from build123d import *

# Parameters (mm, degrees)
SKETCH2_R                  = 5.5499
BOSS_EXTRUDE1_DEPTH        = 3.175
CUT_EXTRUDE1_DEPTH         = 3.175
CUT_EXTRUDE6_DEPTH         = 331.886967859
CUT_EXTRUDE6_DEPTH_BACK    = 331.886967859
SKETCH32_R                 = 2.38125
CUT_EXTRUDE4_DEPTH         = 331.886967859
F_1_1_DIAMETER_HOLE1_D     = 31.75
F_8_CLEARANCE_HOLE1_D      = 4.4958
FILLET1_R                  = 25.4
FILLET2_R                  = 6.35
CUT_EXTRUDE7_START         = -1.74625
SKETCH34_R                 = 3.968749998
SKETCH34_R_2               = 3.96875
SKETCH34_R_3               = 3.968749996
CUT_EXTRUDE7_DEPTH         = 1.74625
F_8_0_199_DIAMETER_HOLE1_D = 5.0546
CUT_EXTRUDE9_DEPTH         = 331.886967859


with BuildPart() as part:
    # Sketch2 → Boss-Extrude1 (new, symmetric)
    with BuildSketch(Plane(origin=(0, 0, 0), x_dir=(0, 0, -1), z_dir=(1, 0, 0))):
        with BuildLine():
            Line((184.861603477, 125.395219788), (192.888179376, 122.398060471))
            ThreePointArc((192.888179376, 122.398060471), (197.134402772, 119.670037319), (199.868014027, 115.427409246))
            ThreePointArc((199.868014027, 115.427409246), (205.79135088, 101.944347228), (213.165326628, 89.196666555))
            ThreePointArc((213.165326628, 89.196666555), (245.495612564, 46.296629776), (283.201634595, 8.035468699))
            ThreePointArc((283.201634595, 8.035468699), (289.498729419, -0.543862964), (291.728224202, -10.95))
            Line((291.728224202, -10.95), (291.728224202, -63.147045251))
            ThreePointArc((291.728224202, -63.147045251), (290.86274019, -69.721048996), (288.325269458, -75.847045251))
            Line((288.325269458, -75.847045251), (279.028224202, -91.949999995))
            Line((279.028224202, -91.949999995), (258.619227522, -91.949999995))
            ThreePointArc((258.619227522, -91.949999995), (257.031727522, -90.362499995), (255.444227522, -91.949999995))
            Line((255.444227522, -91.949999995), (255.444227522, -98.3))
            Line((255.444227522, -98.3), (230.044227522, -98.3))
            Line((230.044227522, -98.3), (230.044227522, -91.949999995))
            ThreePointArc((230.044227522, -91.949999995), (228.456727522, -90.362499995), (226.869227522, -91.949999995))
            Line((226.869227522, -91.949999995), (206.460230842, -91.949999995))
            ThreePointArc((206.460230842, -91.949999995), (203.285230842, -88.774999995), (200.110230842, -91.949999995))
            Line((200.110230842, -91.949999995), (200.110230842, -110.516313332))
            ThreePointArc((200.110230842, -110.516313332), (188.495902289, -129.333888909), (175.117759697, -146.941247574))
            ThreePointArc((175.117759697, -146.941247574), (139.333425556, -150.071971144), (136.202701987, -114.287637002))
            ThreePointArc((136.202701987, -114.287637002), (177.123417321, -15.496291061), (153.979316793, 88.9))
            ThreePointArc((153.979316793, 88.9), (156.586799992, 118.007464254), (184.861603477, 125.395219788))
        make_face()
        with Locations((188.725443767, 111.25)):
            Circle(SKETCH2_R, mode=Mode.SUBTRACT)
    extrude(amount=BOSS_EXTRUDE1_DEPTH, both=True)

    # Sketch4 → Cut-Extrude1 (cut)
    with BuildSketch(Plane.ZY.offset(3.175)):
        with BuildLine():
            ThreePointArc((-142.891227531, -119.899976319), (-139.536446205, -120.193481654), (-139.24294087, -116.838700328))
            ThreePointArc((-139.24294087, -116.838700328), (-180.470281158, -21.687694559), (-162.960405636, 80.521951489))
            ThreePointArc((-162.960405636, 80.521951489), (-164.040385384, 83.711676692), (-167.230110587, 82.631696943))
            ThreePointArc((-167.230110587, 82.631696943), (-185.19876014, -22.255931098), (-142.891227531, -119.899976319))
        make_face()
    extrude(amount=-CUT_EXTRUDE1_DEPTH, mode=Mode.SUBTRACT)

    # Sketch32 → Cut-Extrude6 (cut, two sides: drawn at the far end of the back side and taken through both)
    with BuildSketch(Plane.ZY.offset(3.175).offset(-CUT_EXTRUDE6_DEPTH_BACK)):
        with Locations((-159.478578107, 92.075)):
            Circle(SKETCH32_R)
    extrude(amount=CUT_EXTRUDE6_DEPTH + CUT_EXTRUDE6_DEPTH_BACK, mode=Mode.SUBTRACT)

    # Sketch23 → Cut-Extrude4 (cut, through all)
    with BuildSketch(Plane(origin=(3.175, 0, 0), x_dir=(0, 0, -1), z_dir=(1, 0, 0))):
        with BuildLine():
            Line((191.834020078, -91.95), (191.834020078, -98.3))
            ThreePointArc((191.834020078, -98.3), (190.246520078, -99.8875), (188.659020078, -98.3))
            Line((188.659020078, -98.3), (175.959020078, -98.3))
            ThreePointArc((175.959020078, -98.3), (174.371520078, -99.8875), (172.784020078, -98.3))
            Line((172.784020078, -98.3), (172.784020078, -91.95))
            ThreePointArc((172.784020078, -91.95), (174.371520078, -90.3625), (175.959020078, -91.95))
            Line((175.959020078, -91.95), (188.659020078, -91.95))
            ThreePointArc((188.659020078, -91.95), (190.246520078, -90.3625), (191.834020078, -91.95))
        make_face()
    extrude(amount=-CUT_EXTRUDE4_DEPTH, mode=Mode.SUBTRACT)

    # 1 (1) Diameter Hole1 (through all)
    with Locations(Plane(origin=(3.175, 0, 0), x_dir=(0, 0, -1), z_dir=(1, 0, 0))):
        with Locations((255.178224202, -28.45)):
            Hole(F_1_1_DIAMETER_HOLE1_D / 2)

    # #8 Clearance Hole1 (through all)
    with Locations(Plane.ZY.offset(3.175)):
        with Locations((-273.138736444, -46.410512242), (-237.21771196, -10.489487758)):
            Hole(F_8_CLEARANCE_HOLE1_D / 2)

    # Fillet1
    fillet1_edges = [part.edges().sort_by_distance(p)[0] for p in [
        (0, -110.516313332, -200.110230842),
    ]]
    fillet(fillet1_edges, radius=FILLET1_R)

    # Fillet2
    fillet2_edges = [part.edges().sort_by_distance(p)[0] for p in [
        (0, -91.949999995, -206.460230842),
    ]]
    fillet(fillet2_edges, radius=FILLET2_R)

    # Sketch34 → Cut-Extrude7 (cut)
    with BuildSketch(Plane.ZY.offset(3.175).offset(CUT_EXTRUDE7_START)):
        with Locations((-272.678224202, -72.899999995)):
            Circle(SKETCH34_R)
        with Locations((-272.678224202, 3.300000005)):
            Circle(SKETCH34_R)
        with Locations((-209.953929472, -72.899999995)):
            Circle(SKETCH34_R_2)
        with Locations((-221.091752478, 22.660527049)):
            Circle(SKETCH34_R)
        with Locations((-200.007931611, 96.911762922)):
            Circle(SKETCH34_R_3)
        with Locations((-152.402488977, -139.565014501)):
            Circle(SKETCH34_R_2)
    extrude(amount=CUT_EXTRUDE7_DEPTH, mode=Mode.SUBTRACT)

    # #8 (0.199) Diameter Hole1 (through all)
    with Locations(Plane(origin=(3.175, 0, 0), x_dir=(0, 0, -1), z_dir=(1, 0, 0))):
        with Locations((272.678224202, -72.899999995), (209.953929472, -72.899999995), (221.091752478, 22.660527049), (200.007931611, 96.911762922), (272.678224202, 3.300000005), (152.402488977, -139.565014501)):
            Hole(F_8_0_199_DIAMETER_HOLE1_D / 2)

    # Sketch38 → Cut-Extrude9 (cut, through all)
    with BuildSketch(Plane(origin=(3.175, 0, 0), x_dir=(0, 0, -1), z_dir=(1, 0, 0))):
        with BuildLine():
            Line((205.914798647, 28.562805507), (224.924360785, 39.537981324))
            ThreePointArc((224.924360785, 39.537981324), (227.99131211, 43.870819192), (226.69603004, 49.018820627))
            ThreePointArc((226.69603004, 49.018820627), (214.944800076, 64.327050851), (203.910748393, 80.160023463))
            ThreePointArc((203.910748393, 80.160023463), (190.936466062, 83.542932982), (186.142659774, 71.021131989))
            ThreePointArc((186.142659774, 71.021131989), (192.251844092, 52.271592857), (196.477565484, 33.009956649))
            ThreePointArc((196.477565484, 33.009956649), (200.032947992, 28.317899385), (205.914798647, 28.562805507))
        make_face()
        with BuildLine():
            Line((205.310000647, -4.207176979), (211.8854012, -4.207176979))
            ThreePointArc((211.8854012, -4.207176979), (216.375529261, -6.067048919), (218.2354012, -10.557176979))
            Line((218.2354012, -10.557176979), (218.2354012, -46.34282301))
            ThreePointArc((218.2354012, -46.34282301), (216.375529261, -50.832951071), (211.8854012, -52.69282301))
            Line((211.8854012, -52.69282301), (200.289772847, -52.69282301))
            ThreePointArc((200.289772847, -52.69282301), (195.319253016, -50.294586238), (194.103216157, -44.911384462))
            ThreePointArc((194.103216157, -44.911384462), (197.299266335, -27.67833955), (198.968379006, -10.23108657))
            ThreePointArc((198.968379006, -10.23108657), (200.936682347, -5.953201844), (205.310000647, -4.207176979))
        make_face()
        with BuildLine():
            Line((229.003929472, -65.39282301), (253.628224202, -65.39282301))
            ThreePointArc((253.628224202, -65.39282301), (258.118352263, -67.25269495), (259.978224202, -71.74282301))
            Line((259.978224202, -71.74282301), (259.978224202, -72.899999995))
            ThreePointArc((259.978224202, -72.899999995), (258.118352263, -77.390128055), (253.628224202, -79.249999995))
            Line((253.628224202, -79.249999995), (229.003929472, -79.249999995))
            ThreePointArc((229.003929472, -79.249999995), (224.513801412, -77.390128055), (222.653929472, -72.899999995))
            Line((222.653929472, -72.899999995), (222.653929472, -71.74282301))
            ThreePointArc((222.653929472, -71.74282301), (224.513801412, -67.25269495), (229.003929472, -65.39282301))
        make_face()
        with BuildLine():
            Line((178.614385619, -107.825), (163.596957108, -107.825))
            ThreePointArc((163.596957108, -107.825), (157.868812502, -109.190170518), (153.372147289, -112.9921875))
            ThreePointArc((153.372147289, -112.9921875), (151.919142792, -114.938348924), (150.441444733, -116.865827797))
            ThreePointArc((150.441444733, -116.865827797), (149.54669032, -123.085290269), (154.438269364, -127.02924176))
            ThreePointArc((154.438269364, -127.02924176), (158.545587593, -128.449604505), (161.93353243, -131.171611694))
            ThreePointArc((161.93353243, -131.171611694), (166.924642658, -133.320901925), (171.750540646, -130.822634844))
            ThreePointArc((171.750540646, -130.822634844), (177.370609198, -123.095397934), (182.643281535, -115.127067669))
            ThreePointArc((182.643281535, -115.127067669), (182.784283536, -110.2867702), (178.614385619, -107.825))
        make_face()
        with BuildLine():
            ThreePointArc((229.352144485, 13.013977205), (232.770157357, 17.670050169), (233.772565242, 23.358372055))
            ThreePointArc((233.772565242, 23.358372055), (237.643482483, 29.557433307), (244.785557135, 28.00722998))
            ThreePointArc((244.785557135, 28.00722998), (250.350507009, 22.07652944), (256.029490766, 16.254930046))
            ThreePointArc((256.029490766, 16.254930046), (257.782536544, 10.684174236), (254.244609375, 6.037717399))
            ThreePointArc((254.244609375, 6.037717399), (245.943574881, 3.17910276), (237.21771196, 2.210512242))
            ThreePointArc((237.21771196, 2.210512242), (235.966501016, 2.148726957), (234.727464312, 1.96397227))
            ThreePointArc((234.727464312, 1.96397227), (227.77212485, 5.41294467), (229.352144485, 13.013977205))
        make_face()
    extrude(amount=-CUT_EXTRUDE9_DEPTH, mode=Mode.SUBTRACT)


solid = part.part
Source: CAD feature listing. Evaluate the final solid. Frame: model axes, mm. A direction names the side the tool comes from. Round coordinates to 2 decimals unless told otherwise and drop trailing zeros. Order: outer loops, then holes, each group sorted by start corner. A loop starts at its lowest first (then second) coordinate and runs counter-clockwise, first axis right, second up. Notation, with made-up numbers: (74, -33) -> (92, -33) arc R15 cw to (92, -29) -> close; hole circle Ø4 at (0.25, -37.5). An arc over 180 degrees is marked (long way). Answer as CSV lines item,"result".
Item 1: Section D-D, the plane x = 2. Count the separate pieces of the cut face and the enclosed holes in it, plus the area to 3 significant figures.
A:
separate pieces,"1"
enclosed holes,"17"
area,"18,000 mm²"
Item 2: Section C-C, the plane y = 111.25. Return loops of the section in (x, z) (3 decimals), plus the area to 3 significant figures.
A:
outline,"(-3.175, -201.515) -> (3.175, -201.515) -> (3.175, -194.275) -> (-3.175, -194.275) -> close; (-3.175, -183.176) -> (3.175, -183.176) -> (3.175, -152.481) -> (-3.175, -152.481) -> close"
area,"241 mm²"
Item 3: Line query: L1, parallel to Y at x = -1.75, z = -226; L2, parallel to Y at x = 0.75, z = -153; L3, parallel to Y at x = 3, z = -241. Output: solid intervals per line, ascending.
A:
L1,"-91.95 to -78.49, -66.15 to 40.32, 49.89 to 70.73"
L2,"-155.87 to -142.02, -137.11 to -126.62, -113.5 to -90.58, 90.77 to 112.43"
L3,"-98.3 to -79.25, -65.39 to -35.59, -21.31 to 2.39, 30 to 51.6"
Item 4: Reachability of faces 4 (the face through (0.04, 46.87, -245)), 5 (the face through (0.04, -77.34, -258.17)), 6 (the face through (-2.29, -71.71, -268.89)) from +Z, -Z, +X, -X, +Y, -Y: full face, straight path, thin tool, end or side. Return the list, or none.
A:
face 4,"-Z, +X, -X, +Y"
face 5,"+X, -X"
face 6,"-X"
Item 5: Section A-A, the plane y = 60. Return loops of the section in (x, z) (3 decimals).
A:
outline,"(-3.175, -234.184) -> (3.175, -234.184) -> (3.175, -218.154) -> (-3.175, -218.154) -> close; (-3.175, -189.982) -> (3.175, -189.982) -> (3.175, -167.37) -> (-3.175, -167.37) -> (-3.175, -171.581) -> (0, -171.581) -> (0, -176.618) -> (-3.175, -176.618) -> close"
Item 6: Pin query (flat end, axial travel): pin 1 Ø6.5 at (y, z) = (-72.9, -209.95) entering from -X; pin 2 Ø2 at (x, z) = (1.5, -227.5) entering from -Y; pin 3 Ø0.9 at (x, y) = (-1.5, -72) entering from -Z; pin 4 Ø10.5 at (y, z) = (3.3, -272.68) entering from -X (3 decimals). Return the tip coordinate at first contact, or that it passes through.
A:
pin 1,"x = -1.43"
pin 2,"y = -91.95"
pin 3,"z = -290.3"
pin 4,"x = -3.175"
Item 7: Pull-direction query (Z, two-part tool) for faces 1 (the face through (0.04, -0.41, -289.44)), 2 (the face through (-1.61, -20.755, -185.373)), 3 (the face through (-2.29, 21.14, -217.426)); classes: pulls with the +Z half, pulls with the -Z half, needs draft (parallel to the pull), parting line crosses it, or undercut.
A:
face 1,"pulls with the -Z half"
face 2,"undercut"
face 3,"undercut"
Item 8: Section B-B, the plane y = -34. Return loops of the section in (x, z) (3 decimals).
A:
outline,"(-3.175, -291.728) -> (3.175, -291.728) -> (3.175, -270.051) -> (-3.175, -270.051) -> close; (-3.175, -240.305) -> (3.175, -240.305) -> (3.175, -218.235) -> (-3.175, -218.235) -> close; (-3.175, -196.309) -> (3.175, -196.309) -> (3.175, -174.519) -> (-3.175, -174.519) -> (-3.175, -178.561) -> (0, -178.561) -> (0, -183.406) -> (-3.175, -183.406) -> close"
